Source: CAD feature listing. Evaluate the final solid. Frame: model axes, mm. Give positions to 0.01 mm unless a question says otherwise; leave off trailing zeros. Loops run counter-clockwise (first coordinate to the right, second up) from the corner with the lowest first, then second, coordinate; pieces in that order, holes last. Notation, with made-up numbers: M 6.5,6 L 46.5,6 A21 cw 46.5,25 Z; hole C 30.25,73.25 d11. An arc over 180 degrees is marked long. Answer in a Markdown table with one row per item.
```python
from build123d import *

# Parameters (mm, degrees)
F0_W     = 159
F0_H     = 134
F0_W_2   = 16
F0_H_2   = 16
F0_W_3   = 91
F1_DEPTH = 10
F2_W     = 159
F2_H     = 134
F3_DEPTH = 2


with BuildPart() as f1:
    # F0 (on Top) → F1 (new body)
    with BuildSketch(Plane.XY):
        Rectangle(F0_W, F0_H)
        with Locations((-62.5, -50)):
            Rectangle(F0_W_2, F0_H_2, mode=Mode.SUBTRACT)
        with Locations((-37.5, -50)):
            Rectangle(F0_W_2, F0_H_2, mode=Mode.SUBTRACT)
        with Locations((-12.5, -50)):
            Rectangle(F0_W_2, F0_H_2, mode=Mode.SUBTRACT)
        with Locations((-62.5, -25)):
            Rectangle(F0_W_2, F0_H_2, mode=Mode.SUBTRACT)
        with Locations((-37.5, -25)):
            Rectangle(F0_W_2, F0_H_2, mode=Mode.SUBTRACT)
        with Locations((-12.5, -25)):
            Rectangle(F0_W_2, F0_H_2, mode=Mode.SUBTRACT)
        with Locations((12.5, -50)):
            Rectangle(F0_W_2, F0_H_2, mode=Mode.SUBTRACT)
        with Locations((37.5, -50)):
            Rectangle(F0_W_2, F0_H_2, mode=Mode.SUBTRACT)
        with Locations((62.5, -50)):
            Rectangle(F0_W_2, F0_H_2, mode=Mode.SUBTRACT)
        with Locations((12.5, -25)):
            Rectangle(F0_W_2, F0_H_2, mode=Mode.SUBTRACT)
        with Locations((37.5, -25)):
            Rectangle(F0_W_2, F0_H_2, mode=Mode.SUBTRACT)
        with Locations((62.5, -25)):
            Rectangle(F0_W_2, F0_H_2, mode=Mode.SUBTRACT)
        with Locations((-62.5, 0)):
            Rectangle(F0_W_2, F0_H_2, mode=Mode.SUBTRACT)
        with Locations((-62.5, 25)):
            Rectangle(F0_W_2, F0_H_2, mode=Mode.SUBTRACT)
        with Locations((-37.5, 25)):
            Rectangle(F0_W_2, F0_H_2, mode=Mode.SUBTRACT)
        with Locations((-12.5, 25)):
            Rectangle(F0_W_2, F0_H_2, mode=Mode.SUBTRACT)
        with Locations((-62.5, 50)):
            Rectangle(F0_W_2, F0_H_2, mode=Mode.SUBTRACT)
        with Locations((-37.5, 50)):
            Rectangle(F0_W_2, F0_H_2, mode=Mode.SUBTRACT)
        with Locations((-12.5, 50)):
            Rectangle(F0_W_2, F0_H_2, mode=Mode.SUBTRACT)
        Rectangle(F0_W_3, F0_H_2, mode=Mode.SUBTRACT)
        with Locations((12.5, 25)):
            Rectangle(F0_W_2, F0_H_2, mode=Mode.SUBTRACT)
        with Locations((37.5, 25)):
            Rectangle(F0_W_2, F0_H_2, mode=Mode.SUBTRACT)
        with Locations((62.5, 0)):
            Rectangle(F0_W_2, F0_H_2, mode=Mode.SUBTRACT)
        with Locations((62.5, 25)):
            Rectangle(F0_W_2, F0_H_2, mode=Mode.SUBTRACT)
        with Locations((12.5, 50)):
            Rectangle(F0_W_2, F0_H_2, mode=Mode.SUBTRACT)
        with Locations((37.5, 50)):
            Rectangle(F0_W_2, F0_H_2, mode=Mode.SUBTRACT)
        with Locations((62.5, 50)):
            Rectangle(F0_W_2, F0_H_2, mode=Mode.SUBTRACT)
    extrude(amount=F1_DEPTH)

    # F2 (on face) → F3 (join)
    with BuildSketch(Plane(origin=(0, 0, 0), x_dir=(1, 0, 0), z_dir=(0, 0, -1))):
        Rectangle(F2_W, F2_H)
    extrude(amount=F3_DEPTH)


solid = f1.part
```
1) Pin query (flat end, axial travel): pin 1 Ø3 at (x, y) = (57, -26) entering from +Z. Return the tip coordinate at first contact, or that it passes through.
Reply:
| item | result |
|---|---|
| pin 1 | stops at z = 0 |
2) Section A-A, the plane y = 0. Return loops of the section in (x, z), then the cut area to 3 significant figures.
Reply:
| item | result |
|---|---|
| outline | M -79.5,-2 L 79.5,-2 L 79.5,10 L 70.5,10 L 70.5,0 L 54.5,0 L 54.5,10 L 45.5,10 L 45.5,0 L -45.5,0 L -45.5,10 L -54.5,10 L -54.5,0 L -70.5,0 L -70.5,10 L -79.5,10 Z |
| area | 678 mm² |
3) Section B-B, the plane x = -64. Return loops of the section in (y, z).
Reply:
| item | result |
|---|---|
| outline | M -67,-2 L 67,-2 L 67,10 L 58,10 L 58,0 L 42,0 L 42,10 L 33,10 L 33,0 L 17,0 L 17,10 L 8,10 L 8,0 L -8,0 L -8,10 L -17,10 L -17,0 L -33,0 L -33,10 L -42,10 L -42,0 L -58,0 L -58,10 L -67,10 Z |
4) Section D-D, the plane y = 56. Return loops of the section in (x, z), then the cut area to 3 significant figures.
Reply:
| item | result |
|---|---|
| outline | M -79.5,-2 L 79.5,-2 L 79.5,10 L 70.5,10 L 70.5,0 L 54.5,0 L 54.5,10 L 45.5,10 L 45.5,0 L 29.5,0 L 29.5,10 L 20.5,10 L 20.5,0 L 4.5,0 L 4.5,10 L -4.5,10 L -4.5,0 L -20.5,0 L -20.5,10 L -29.5,10 L -29.5,0 L -45.5,0 L -45.5,10 L -54.5,10 L -54.5,0 L -70.5,0 L -70.5,10 L -79.5,10 Z |
| area | 948 mm² |
5) Section C-C, the plane z = 6. Count the separate pieces of the cut face and the enclosed holes in it, then the cut area to 3 significant figures.
Reply:
| item | result |
|---|---|
| separate pieces | 1 |
| enclosed holes | 27 |
| area | 13,200 mm² |
6) Material intervals for L1, parallel to Y at x = -15.5, z = 0.5; L2, parallel to X at y = 5.5, z = 5.5; L3, parallel to Y at x = 26, z = 5.5, sorted ascending.
Reply:
| item | result |
|---|---|
| L1 | y = -67 to -58, -42 to -33, -17 to -8, 8 to 17, 33 to 42, 58 to 67 |
| L2 | x = -79.5 to -70.5, -54.5 to -45.5, 45.5 to 54.5, 70.5 to 79.5 |
| L3 | y = -67 to -8, 8 to 67 |
